Geometry check sheet. Reference: the model listing, model coordinates, mm. Face numbers are marked on the shaded views. A direction names the side the tool comes from. Round coordinates to 2 decimals unless told otherwise and drop trailing zeros. Write each loop counter-clockwise with the first axis right and the second up, starting at its lowest first coordinate (ties: lowest second). Pieces come first, ordered by that corner, then holes. Notation, with made-up numbers: (33, 61) -> (55, 61) arc R16 cw to (55, 74) -> close; hole circle Ø6 at (75.5, -33). An arc over 180 degrees is marked (long way). Put each result on its own line as item: value. Start each with the question number.
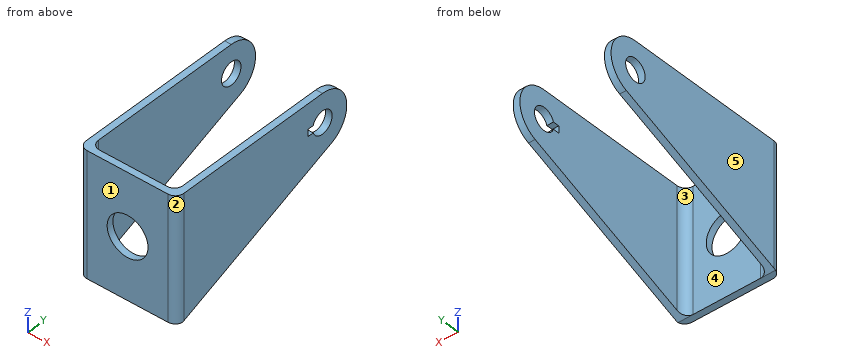
from build123d import *

# Parameters (mm, degrees)
CROQUIS1_R              = 4
SALIENTE_EXTRUIR1_DEPTH = 34.72
CROQUIS2_W              = 30
CROQUIS2_H              = 67.64
CORTAR_EXTRUIR1_DEPTH   = 90.67429063
REDONDEO1_R             = 3
CORTAR_EXTRUIR2_DEPTH   = 89.787215296
CROQUIS4_R              = 7.25
CORTAR_EXTRUIR3_DEPTH   = 88.844453439


with BuildPart() as part:
    # Croquis1 → Saliente-Extruir1 (new body)
    with BuildSketch(Plane(origin=(0, 0, 0), x_dir=(0, 0, -1), z_dir=(1, 0, 0))):
        with BuildLine():
            Line((0, 60), (0, 0))
            Line((0, 0), (44, 0))
            Line((44, 0), (44, 2.36))
            Line((44, 2.36), (19.275687183, 63.736526097))
            ThreePointArc((19.275687183, 63.736526097), (8.096959254, 69.817251953), (0, 60))
        make_face()
        with Locations((10, 60)):
            Circle(CROQUIS1_R, mode=Mode.SUBTRACT)
    extrude(amount=SALIENTE_EXTRUIR1_DEPTH)

    # Croquis2 → Cortar-Extruir1 (cut, through all)
    with BuildSketch(Plane.XY):
        with Locations((17.36, 36.18)):
            Rectangle(CROQUIS2_W, CROQUIS2_H)
    extrude(amount=-CORTAR_EXTRUIR1_DEPTH, mode=Mode.SUBTRACT)

    # Redondeo1
    redondeo1_edges = [part.edges().sort_by_distance(p)[0] for p in [
        (34.72, 0, -22),
        (0, 0, -22),
        (32.36, 2.36, -22),
        (2.36, 2.36, -22),
    ]]
    fillet(redondeo1_edges, radius=REDONDEO1_R)

    # Croquis3 → Cortar-Extruir2 (cut, through all)
    with BuildSketch(Plane.ZY.offset(-32.36)):
        with BuildLine():
            Line((-8.75, 54), (-8.75, 56.200328962))
            ThreePointArc((-8.75, 56.200328962), (-10, 56), (-11.25, 56.200328962))
            Line((-11.25, 56.200328962), (-11.25, 54))
            Line((-11.25, 54), (-8.75, 54))
        make_face()
    extrude(amount=-CORTAR_EXTRUIR2_DEPTH, mode=Mode.SUBTRACT)

    # Croquis4 → Cortar-Extruir3 (cut, through all)
    with BuildSketch(Plane(origin=(0, 2.36, 0), x_dir=(1, 0, 0), z_dir=(0, 1, 0))):
        with Locations(Location((17.36, 22, 0), (0, 0, 270))):
            Circle(CROQUIS4_R)
    extrude(amount=-CORTAR_EXTRUIR3_DEPTH, mode=Mode.SUBTRACT)


solid = part.part
(1) Set-up check for the marked faces 4 and 5: record each of +Z, -Z, +X, -X, +Y, -Y from which the full face is reachable in a straight line by a thin tool's end or side.
(2) Sectioned sample at D-D (z = -17.5). Record the cut outline in (x, y), and give its area (3 significant figures).
(3) Sectioned sample at C-C (y = 22). Record the cut outline in (x, z).
(4) Sectioned sample at A-A (x = 17.36). Record the cut outline in (y, z), and give its area (3 significant figures).
(5) Sectioned sample at B-B (z = -10). Record the cut outline in (x, y).
(6) Material ranges on L1, parallel to X at y = 29, z = -2; L2, parallel to X at y = 3.5, z = -27; L3, parallel to Y at x = 19, z = -4.5, recorded low to high. Write a range as from..to.
(7) Mould release check, pull along X, two halves, no side actions. Record for the marked faces 1, 2 and 3: +X half, -X half, draft (parallel to the pull), parting line (faces both ways), or undercut.
(8) Go/stop test with flat-tipped pins: pin 1 Ø7 at (y, z) = (60, -10) entering from -X; pin 2 Ø4 at (x, z) = (7.5, -20.5) entering from +Y; pin 3 Ø1.8 at (x, y) = (33.5, 55) entering from -Z. Record where each tip stops, or that it passes through.
Found:
1. face 4: +Z, -Z, +Y
1. face 5: +Z, -Z, -X, +Y, -Y
2. outline: (0, 3) arc R3 ccw to (3, 0) -> (11.68, 0) -> (11.68, 2.36) -> (5.36, 2.36) arc R3 cw to (2.36, 5.36) -> (2.36, 66.61) -> (0, 66.61) -> close; (23.04, 0) -> (31.72, 0) arc R3 ccw to (34.72, 3) -> (34.72, 66.61) -> (32.36, 66.61) -> (32.36, 5.36) arc R3 cw to (29.36, 2.36) -> (23.04, 2.36) -> close
2. area: 358 mm2
3. outline: (0, -36.09) -> (2.36, -36.09) -> (2.36, 0) -> (0, 0) -> close; (32.36, -36.09) -> (34.72, -36.09) -> (34.72, 0) -> (32.36, 0) -> close
4. outline: (0, -44) -> (2.36, -44) -> (2.36, -29.25) -> (0, -29.25) -> close; (0, -14.75) -> (2.36, -14.75) -> (2.36, 0) -> (0, 0) -> close
4. area: 69.6 mm2
5. outline: (0, 3) arc R3 ccw to (3, 0) -> (31.72, 0) arc R3 ccw to (34.72, 3) -> (34.72, 54) -> (32.36, 54) -> (32.36, 5.36) arc R3 cw to (29.36, 2.36) -> (5.36, 2.36) arc R3 cw to (2.36, 5.36) -> (2.36, 56) -> (0, 56) -> close; (0, 64) -> (2.36, 64) -> (2.36, 70) -> (0, 70) -> close; (32.36, 64) -> (34.72, 64) -> (34.72, 70) -> (32.36, 70) -> close
6. L1: 0..2.36, 32.36..34.72
6. L2: 0..3.01, 31.71..34.72
6. L3: 0..2.36
7. face 1: draft
7. face 2: +X half
7. face 3: undercut
8. pin 1: through
8. pin 2: y = 2.36
8. pin 3: z = -23.16
